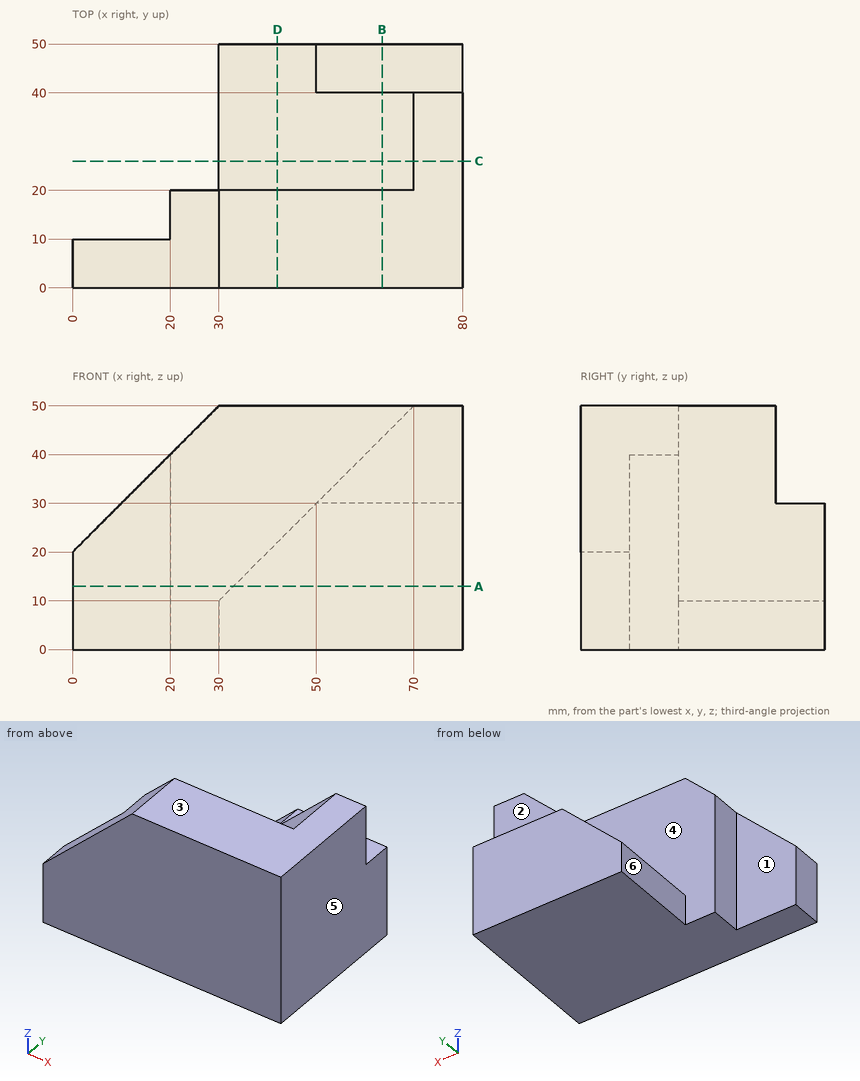
Input: dimensioned drawing with shaded views. Units: mm. Origin: part minimum x, y, z. A direction names the side the tool comes from. Coordinates: 2 decimals unless noted, no trailing zeros. Order: outer loops, then holes, each group sorted by start corner. A loop starts at its lowest first (then second) coordinate and runs counter-clockwise, first axis right, second up. Notation, with made-up numbers: (-29, -14.75) - (-2, -14.75) arc R29 cw to (-2, 12.25) - close; hole circle Ø9 at (25.5, 31.25). An arc over 180 degrees is marked (long way). Return JSON: item names as keys, results as strings. Group by question number.
1. Cut plane B-B (x = 63.5). Output: boundary loops of the cut face in (y, z).
2. Set-up query: the marked faces 1, 2 and 3. Return all of +Z, -Z, +X, -X, +Y, -Y with unobstructed straight access to the full face (end or side cutting, diameter ignored); none if empty.
3. Cut plane C-C (y = 26). Output: boundary loops of the cut face in (x, z).
4. Pin query (flat end, axial travel): pin 1 (1.5 mm diameter, centred on y = 12, z = 5.5, fed in from -X); pin 2 (12 mm diameter, centred on x = 71, y = 31.5, fed in from -Z); pin 3 (1.5 mm diameter, centred on x = 21, z = 33.5, fed in from +Y); pin 4 (5 mm diameter, centred on y = 39, z = 3, fed in from -X). Return the tip coordinate at first contact, or that it passes through.
5. Cut plane A-A (z = 13). Output: boundary loops of the cut face in (x, y).
6. Cut plane D-D (x = 42). Output: boundary loops of the cut face in (y, z), plus the area to 3 significant figures.
7. Material intervals for line 1 along X through (y, z) = (14.5, 15); line 2 along Y through (x, z) = (73, 32.5); line 3 along Y through (x, z) = (34, 34.5), sorted ascending. Write a range as [from, to].
8. Pull-direction query (X, two-part tool) for the marked faces 4, 5 and 6; classes: pulls with the +X half, pulls with the -X half, needs draft (parallel to the pull), parting line crosses it, or undercut.
Resolved:
{
 "1": {"outline": "(0, 0) - (50, 0) - (50, 30) - (40, 30) - (40, 43.5) - (20, 43.5) - (20, 50) - (0, 50) - close"},
 "2": {"face 1": "+Z, -Z, -X, +Y", "face 2": "+Z, +X, -X, +Y", "face 3": "+Z, +X, -X, +Y, -Y"},
 "3": {"outline": "(30, 0) - (80, 0) - (80, 50) - (70, 50) - (30, 10) - close"},
 "4": {"pin 1": "stops at x = 20", "pin 2": "stops at z = 0", "pin 3": "stops at y = 20", "pin 4": "stops at x = 30"},
 "5": {"outline": "(0, 0) - (80, 0) - (80, 50) - (33, 50) - (33, 20) - (20, 20) - (20, 10) - (0, 10) - close"},
 "6": {"outline": "(0, 0) - (50, 0) - (50, 22) - (20, 22) - (20, 50) - (0, 50) - close", "area": "1,660 mm²"},
 "7": {"line 1": "x = [20, 80]", "line 2": "y = [0, 40]", "line 3": "y = [0, 20]"},
 "8": {"face 4": "needs draft", "face 5": "pulls with the +X half", "face 6": "pulls with the -X half"}
}
